Read the model definition and answer for the solid it produces. Units are mm, in the model's axes. A direction names the side the tool comes from. Give positions to 0.01 mm unless a question says otherwise; leave off trailing zeros. Write each loop counter-clockwise with the first axis right and the second up, starting at its lowest first coordinate (ties: lowest second). Pieces come first, ordered by that corner, then holes. Notation, with made-up numbers: M 47,-15.5 L 55,-15.5 A8 cw 55,-5.5 Z; hole C -2,-3 d6. An arc over 180 degrees is marked long. Put each result on its own line as item: value.
from build123d import *

# Parameters (mm, degrees)
SKETCH1_W           = 13
SKETCH1_H           = 22
BOSS_EXTRUDE1_DEPTH = 25
SKETCH2_R           = 3
BOSS_EXTRUDE2_DEPTH = 2
SKETCH3_R           = 2.5
BOSS_EXTRUDE3_DEPTH = 4


with BuildPart() as part:
    # Sketch1 → Boss-Extrude1 (new body)
    with BuildSketch(Plane.XY):
        Rectangle(SKETCH1_W, SKETCH1_H)
    extrude(amount=BOSS_EXTRUDE1_DEPTH)

    # Sketch2 → Boss-Extrude2 (add)
    with BuildSketch(Plane.XY.offset(25)):
        with Locations((0, 7)):
            Circle(SKETCH2_R)
    extrude(amount=BOSS_EXTRUDE2_DEPTH)

    # Sketch3 → Boss-Extrude3 (add)
    with BuildSketch(Plane.XY.offset(27)):
        with Locations((0, 7)):
            Circle(SKETCH3_R)
    extrude(amount=BOSS_EXTRUDE3_DEPTH)


solid = part.part
(1) Section D-D on x = 4 is taken. Determine the outline of the cut face in (y, z).
Result:
outline: M -11,0 L 11,0 L 11,25 L -11,25 Z
(2) Section B-B on y = 7 is taken. Determine the outline of the cut face in (x, z), and give its area (3 significant figures).
Result:
outline: M -6.5,0 L 6.5,0 L 6.5,25 L 3,25 L 3,27 L 2.5,27 L 2.5,31 L -2.5,31 L -2.5,27 L -3,27 L -3,25 L -6.5,25 Z
area: 357 mm²
(3) Straight lines are drawn through the part: line 1 along Z through (x, y) = (-1.25, -4.25); line 2 along Y through (x, z) = (-0.75, 27.5). For each, find the intervals that lie inside material, in ascending order. Write a range as from..to.
Result:
line 1: z = 0..25
line 2: y = 4.62..9.38
(4) Which of the six approach directions +Z, -Z, +X, -X, +Y, -Y give full straight-line access (tool end or side, diameter ignored) to faces 1 (the face through (-6.5, 0, 12)), 2 (the face through (-3, 7, 26))?
Result:
face 1: +Z, -Z, -X, +Y, -Y
face 2: +Z
(5) Given pin 1 Ø4 at (x, y) = (2, -2.5) entering from +Z, flat-ended and moving along its own axis, determine where the tip first touches the part or whether it passes through.
Result:
pin 1: stops at z = 25
(6) Section C-C on z = 26.5 is taken. Determine the outline of the cut face in (x, y), and give its area (3 significant figures).
Result:
outline: C 0,7 d6
area: 28.3 mm²
(7) Section A-A on x = 0 is taken. Determine the outline of the cut face in (y, z).
Result:
outline: M -11,0 L 11,0 L 11,25 L 10,25 L 10,27 L 9.5,27 L 9.5,31 L 4.5,31 L 4.5,27 L 4,27 L 4,25 L -11,25 Z
